Input: dimensioned drawing with shaded views. Units: mm. Origin: part minimum x, y, z. A direction names the side the tool comes from. Round coordinates to 2 decimals unless told otherwise and drop trailing zeros. Loops run counter-clockwise (first coordinate to the right, second up) from the corner with the lowest first, then second, coordinate; pieces in that order, holes last. Notation, with made-up numbers: (0, 56) - (5, 56) arc R14 cw to (5, 82) - close; hole circle Ø10 at (84.5, 74.25). An arc over 180 degrees is marked (long way). One line per question, with ' | ' between items. Start each with the question number.
1. Access query for the marked faces 1, 2 and 3. Directions: +Z, -Z, +X, -X, +Y, -Y. A direction counts if a zero-diameter tool reaches every point of the face in a straight line with its end or side. Return the directions, or none.
2. Ray query, line 1 (Z direction, x = 10, y = 45.5); line 2 (X direction, y = 3, z = 23.5); line 3 (X direction, y = 23.5, z = 3) (1 decimal). Return the intervals inside material, ascending.
3. Cut plane B-B (x = 10.5). Return loops of the section in (y, z), then the cut area to 3 significant figures.
4. Cut plane D-D (z = 7.5). Return loops of the section in (x, y) (1 decimal).
5. Pin query (flat end, axial travel): pin 1 (6.5 mm diameter, centred on x = 54.5, y = 21, fed in from -Z); pin 2 (1 mm diameter, centred on x = 50, y = 15.5, fed in from -Z); pin 3 (10 mm diameter, centred on x = 25, z = 6, fed in from +Y); pin 4 (23 mm diameter, centred on x = 24.37, z = 39.71, fed in from +Y). Return the tip coordinate at first contact, or that it passes through.
6. Cut plane A-A (x = 26.5). Return loops of the section in (y, z).
7. Cut plane C-C (y = 42.5). Return loops of the section in (x, z).
8. Mould query, pull axis Z, two halves, no side actions, for the marked faces 4, 5, 6 and 7. Classes: pulls with the +Z half, pulls with the -Z half, needs draft (parallel to the pull), parting line crosses it, or undercut.
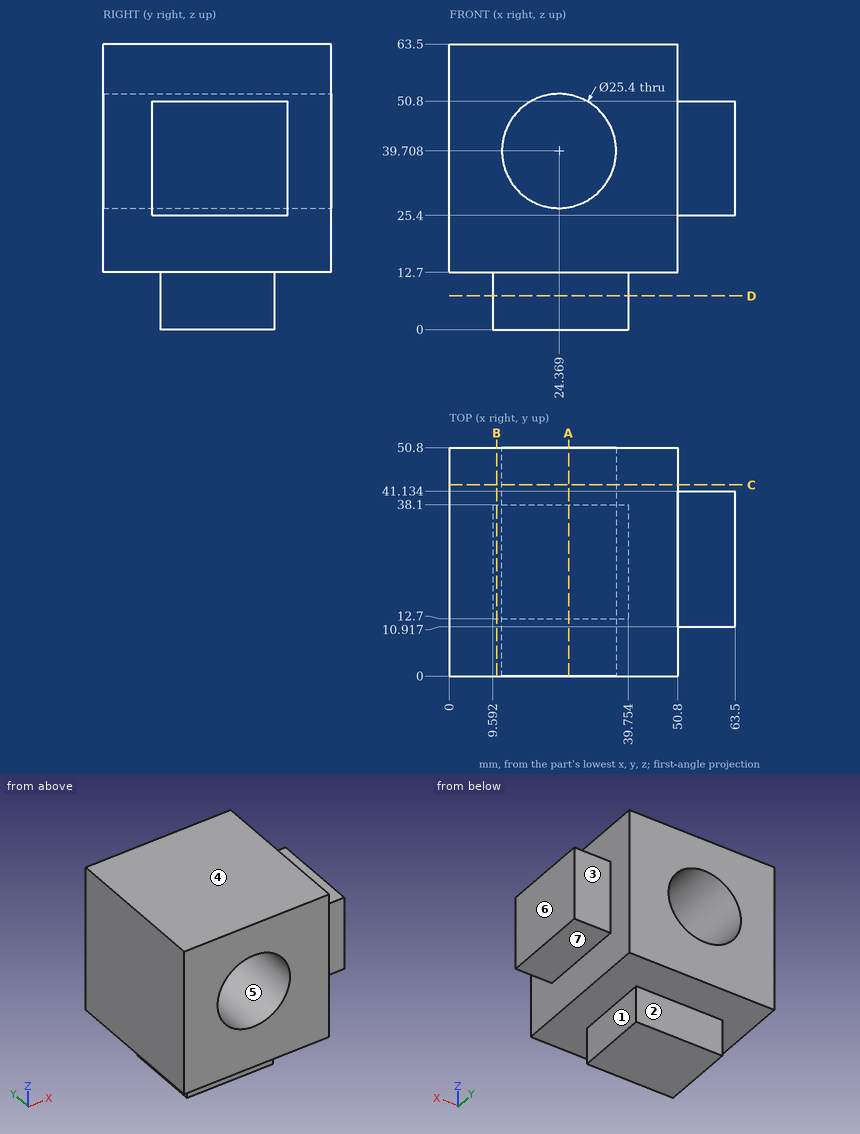
Answers follow:
1) face 1: -Z, +X, +Y, -Y | face 2: -Z, +X, -X, +Y | face 3: +Z, -Z, +X, +Y
2) line 1: z = 12.7 to 63.5 | line 2: x = 0 to 50.8 | line 3: x = 9.6 to 39.8
3) outline: (0, 12.7) - (12.7, 12.7) - (12.7, 0) - (38.1, 0) - (38.1, 12.7) - (50.8, 12.7) - (50.8, 63.5) - (0, 63.5) - close | area: 2,900 mm2
4) outline: (9.6, 12.7) - (39.8, 12.7) - (39.8, 38.1) - (9.6, 38.1) - close
5) pin 1: stops at z = 25.4 | pin 2: stops at z = 12.7 | pin 3: stops at y = 38.1 | pin 4: passes through
6) outline: (0, 12.7) - (12.7, 12.7) - (12.7, 0) - (38.1, 0) - (38.1, 12.7) - (50.8, 12.7) - (50.8, 27.19) - (0, 27.19) - close; (0, 52.23) - (50.8, 52.23) - (50.8, 63.5) - (0, 63.5) - close
7) outline: (0, 12.7) - (50.8, 12.7) - (50.8, 63.5) - (0, 63.5) - close; hole circle Ø25.4 at (24.37, 39.71)
8) face 4: pulls with the +Z half | face 5: undercut | face 6: needs draft | face 7: pulls with the -Z half
